```python
from build123d import *

# Parameters (mm, degrees)
F2_DEPTH = 10


with BuildPart() as f2:
    # F0 (on Front) → F2 (new body)
    with BuildSketch(Plane.XZ):
        Polygon((3.942324, 62.661439), (-3.942324, 62.661439), (-11.764798, 61.673231), (-19.401734, 59.712399), (-26.732694, 56.809867), (-33.642063, 53.011409), (-40.020877, 48.37693), (-45.768537, 42.979517), (-50.7944, 36.904292), (-55.019206, 30.247064), (-58.376325, 23.112822), (-60.812815, 15.614077), (-62.290251, 7.869089), (-62.785332, 0), (-62.290251, -7.869089), (-60.812815, -15.614077), (-58.376325, -23.112822), (-55.019206, -30.247064), (-50.7944, -36.904292), (-45.768537, -42.979517), (-40.020877, -48.37693), (-33.642063, -53.011409), (-26.732694, -56.809867), (-19.401734, -59.712399), (-11.764798, -61.673231), (-3.942324, -62.661439), (3.942324, -62.661439), (11.764798, -61.673231), (19.401734, -59.712399), (26.732694, -56.809867), (33.642063, -53.011409), (40.020877, -48.37693), (45.768537, -42.979517), (50.7944, -36.904292), (55.019206, -30.247064), (58.376325, -23.112822), (60.812815, -15.614077), (62.290251, -7.869089), (62.785332, 0), (62.290251, 7.869089), (60.812815, 15.614077), (58.376325, 23.112822), (55.019206, 30.247064), (50.7944, 36.904292), (45.768537, 42.979517), (40.020877, 48.37693), (33.642063, 53.011409), (26.732694, 56.809867), (19.401734, 59.712399), (11.764798, 61.673231), align=None)
    extrude(amount=F2_DEPTH)


solid = f2.part
```
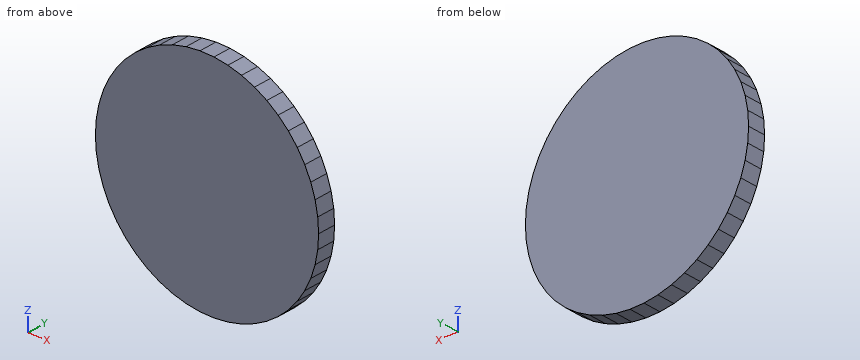
Build history of the part. All positions in model axes, mm. Coordinates: 2 decimals unless noted, no trailing zeros. Order: outer loops, then holes, each group sorted by start corner. A loop starts at its lowest first (then second) coordinate and runs counter-clockwise, first axis right, second up. Notation, with made-up numbers: M -37.75,64.25 L -28.75,64.25 A17 ccw -28.75,81.25 Z; hole C -5,39 d7. An arc over 180 degrees is marked long. One line per question, with ' | ' between items. Start each with the question number.
1. Wall check: line 1 along Z through (x, y) = (-15, -2); line 2 along X through (y, z) = (-5.75, -7.5); line 3 along X through (y, z) = (-1.25, 2). Give the ranges that are in metal, low to high. Write a range as [from, to].
2. Cut at A-A (z = 54.5). Write the cut outline in (x, y), plus the area to 3 significant figures.
3. Cut at B-B (x = -17.5). Write the cut outline in (y, z).
4. Flat gauge pins, fed straight in: P1, Ø4, axis at y = -8, z = 11, coming from the -X side; P2, Ø1.5, axis at y = -7, z = 27, coming from the -X side; P3, Ø4, axis at x = -36, y = -2, coming from the +Z side. Where does each tip first touch, or does it go through?
The answers:
1) line 1: z = [-60.84, 60.84] | line 2: x = [-62.31, 62.31] | line 3: x = [-62.66, 62.66]
2) outline: M -30.93,-10 L 30.93,-10 L 30.93,0 L -30.93,0 Z | area: 619 mm2
3) outline: M -10,-60.2 L 0,-60.2 L 0,60.2 L -10,60.2 Z
4) P1: stops at x = -62.07 | P2: stops at x = -56.9 | P3: stops at z = 52.75
